Autodesk Fusion 360 part; units mm, degrees
sketch "Sketch1" plane through (0, 0, 0) normal (0, 0, 1) x (1, 0, 0)
  circle A0 centre (0, 0) radius 38.0746
  dimension "d1" = 76.1492
extrude "Extrude1" add sketch "Sketch1" along normal blind 3.175
sketch "Sketch2" plane through (0, 0, 3.175) normal (0, 0, 1) x (-1, 0, 0)
  circle A0 centre (0, 0) radius 38.0746
  circle A1 centre (0, 0) radius 36.5125
  dimension "d4" = 73.025
extrude "Extrude2" add sketch "Sketch2" along normal blind 3.175 contours A1
sketch "Sketch3" plane through (0, 0, 6.35) normal (0, 0, 1) x (-1, 0, 0)
  circle A0 centre (0, 0) radius 36.5125
  circle A1 centre (25.4, 0) radius 3.175
  circle A2 centre (-25.4, 0) radius 3.175
  circle A3 centre (0, -7.2644) radius 11.43
  circle A4 centre (0, 20.6756) radius 5.08
  circle A5 centre (0, 0) radius 38.0746
  dimension "d7" = 6.35
  dimension "d8" = 6.35
  dimension "d9" = 50.8
  dimension "d10" = 25.4
  dimension "d11" = 10.16
  dimension "d12" = 20.6756
  dimension "d13" = 22.86
  dimension "d14" = 27.94
extrude "Extrude3" cut sketch "Sketch3" against normal blind 22.86 contours A1 | A2 | A3 | A4
sketch "Sketch4" plane through (0, 0, 6.35) normal (0, 0, 1) x (-1, 0, 0)
  circle A0 centre (-25.4, 0) radius 3.175
  circle A1 centre (0, 20.6756) radius 5.08
  circle A2 centre (0, -7.2644) radius 11.43
  circle A3 centre (25.4, 0) radius 3.175
  circle A4 centre (0, 0) radius 36.5125
  circle A5 centre (15.494, -22.7584) radius 1.4986
  circle A6 centre (15.494, 8.2296) radius 1.4986
  circle A7 centre (-15.494, 8.2296) radius 1.4986
  circle A8 centre (-15.494, -22.7584) radius 1.4986
  dimension "d17" = 2.9972
  dimension "d18" = 30.988
  dimension "d19" = 15.494
  dimension "d20" = 15.494
  dimension "d21" = 30.988
extrude "Extrude4" cut sketch "Sketch4" against normal blind 1.016 contours A5 | A6 | A7 | A8
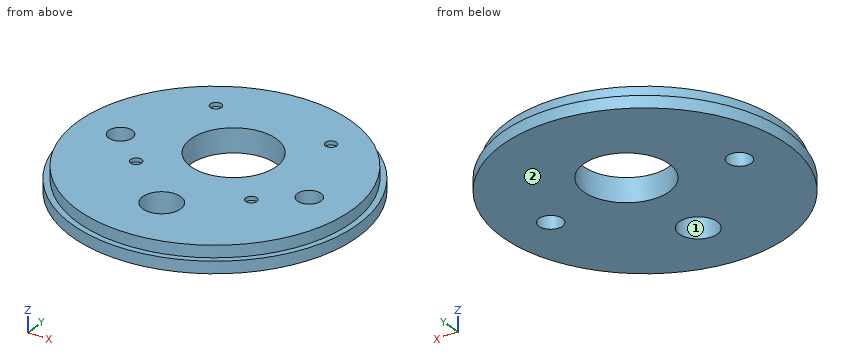
Work out the finished part from the listing and answer in its coordinate system (mm). Face numbers are marked on the shaded views. Coordinates: 2 decimals unless noted, no trailing zeros. Write each loop counter-clockwise with the first axis right and the second up, starting at its lowest first coordinate (ties: lowest second). Pieces come first, ordered by that corner, then holes. Notation, with made-up numbers: (-18.75, 33.25) - (4.25, 33.25) arc R15 cw to (4.25, 49.25) - close; hole circle Ø7 at (9, 19). An arc over 180 degrees is marked (long way). Answer as a JSON object with one key per item and string values.
Q1. Find section D-D (x = 25.4). Write down the section's boundary in (y, z) (3 decimals).
Results list:
{"outline": "(-28.364, 0) - (-3.175, 0) - (-3.175, 6.35) - (-26.23, 6.35) - (-26.23, 3.175) - (-28.364, 3.175) - close; (3.175, 0) - (28.364, 0) - (28.364, 3.175) - (26.23, 3.175) - (26.23, 6.35) - (3.175, 6.35) - close"}
Q2. Find section A-A (x = 0). State how many separate pieces and enclosed holes the cut face has, plus the area to 3 significant figures.
Results list:
{"separate pieces": "3", "enclosed holes": "0", "area": "264 mm^2"}
Q3. Consider L1, parallel to Y at x = 0.5, z = 2.25; L2, parallel to X at y = -1.5, z = 3.5; L3, parallel to Y at x = -2, z = 2.75. Determine where each line is inside the solid, lowest interval first. Write a range as from..to.
Results list:
{"L1": "y = -38.07..-25.73, -15.62..-4.15, 18.68..38.07", "L2": "x = -36.48..-28.2, -22.6..-7.34, 7.34..22.6, 28.2..36.48", "L3": "y = -38.02..-25.35, -16.01..-3.99, 18.52..38.02"}
Q4. For a pull along X with two mould halves and no side action, classify the marked faces 1 and 2 as pulls with the +X half, pulls with the -X half, needs draft (parallel to the pull), parting line crosses it, or undercut.
Results list:
{"face 1": "undercut", "face 2": "needs draft"}
Q5. Given pin 1 Ø5 at (x, y) = (-4, -2) entering from +Z; pin 2 Ø1.5 at (x, y) = (-15, 23) entering from +Z; pin 3 Ø3 at (y, z) = (30, 1) entering from +X, each flat-ended and moving along its own axis, determine where each tip first touches the part or whether it passes through.
Results list:
{"pin 1": "stops at z = 6.35", "pin 2": "stops at z = 5.33", "pin 3": "stops at x = 25.25"}
